Answer from the drawing. Dimensions are ordinates in mm from the lowest x, y and z of the part. Give positions to 0.01 mm unless a question says otherwise; leave off trailing zeros. Loops run counter-clockwise (first coordinate to the right, second up) from the corner with the lowest first, then second, coordinate; pieces in that order, holes last. Notation, with made-up numbers: M -5.75,44.25 L 43.25,44.25 A9 cw 43.25,61.25 Z; hole C 81.5,62 d11. An arc over 180 degrees is marked long. Return JSON: item names as keys, results as strings. Group by question number.
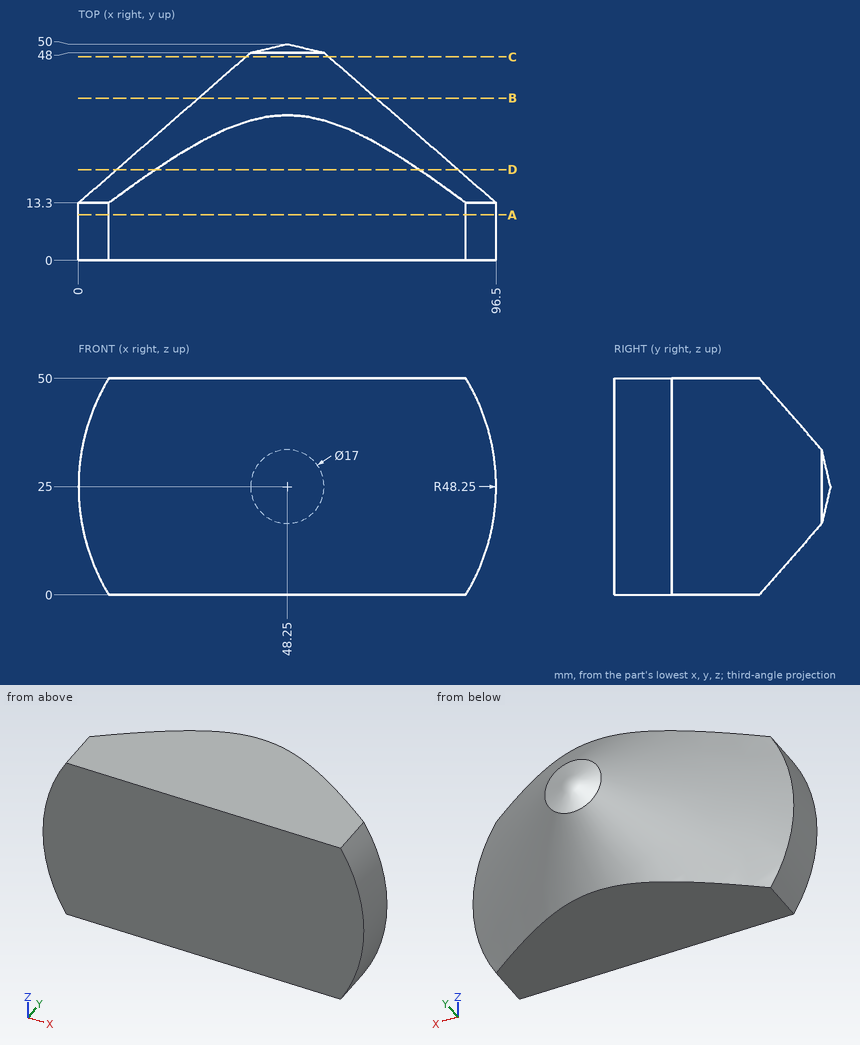
1. Find section D-D (y = 21). Write down the section's boundary in (x, z), and give its area (3 significant figures).
2. Straight lines are drawn through the part: line 1 along X through (y, z) = (6.5, 26); line 2 along Y through (x, z) = (10, 6); line 3 along Y through (x, z) = (84, 25.5). For each, find the intervals that lie inside material, in ascending order.
3. Find section B-B (y = 37.5). Write down the section's boundary in (x, z).
4. Find section C-C (y = 47). Write down the section's boundary in (x, z), and give its area (3 significant figures).
5. Find section A-A (y = 10.5). Write down the section's boundary in (x, z), and give its area (3 significant figures).
6. Flat-ended cylindrical pins translate along their axes: P1, Ø5, axis at x = 19.5, y = 28, coming from the -Z side; P2, Ø10, axis at y = 17, z = 42.5, coming from the -X side; P3, Ø8, axis at x = 55, z = 41, coming from the +Y side. Find the tip coordinate at first contact, or state that the pin passes through.
Result:
{
 "1": {"outline": "M 17.76,0 L 78.74,0 A39.43 ccw 78.74,50 L 17.76,50 A39.43 ccw Z", "area": "3,660 mm2"},
 "2": {"line 1": "x = 0.01 to 96.49", "line 2": "y = 0 to 18.14", "line 3": "y = 0 to 24.21"},
 "3": {"outline": "C 48.25,25 d41.06"},
 "4": {"outline": "C 48.25,25 d19.29", "area": "292 mm2"},
 "5": {"outline": "M 6.98,0 L 89.52,0 A48.25 ccw 89.52,50 L 6.98,50 A48.25 ccw Z", "area": "4,600 mm2"},
 "6": {"P1": "stops at z = 5.17", "P2": "stops at x = 2.12", "P3": "stops at y = 43.75"}
}
